```python
from build123d import *

# Parameters (mm, degrees)
SKIZZE1_W                       = 80
SKIZZE1_H                       = 60
AUFSATZ_LINEAR_AUSTRAGEN1_DEPTH = 10
SKIZZE2_W                       = 80
SKIZZE2_H                       = 10
AUFSATZ_LINEAR_AUSTRAGEN2_DEPTH = 10
SKIZZE3_R                       = 11.35
SCHNITT_LINEAR_AUSTRAGEN1_DEPTH = 2.2
SKIZZE4_R                       = 3
SCHNITT_LINEAR_AUSTRAGEN2_DEPTH = 12.2
SKIZZE5_R                       = 2.25
SCHNITT_LINEAR_AUSTRAGEN3_DEPTH = 12.2
SKIZZE6_R                       = 11
SCHNITT_LINEAR_AUSTRAGEN4_DEPTH = 12.2
SKIZZE7_R                       = 1.6
SCHNITT_LINEAR_AUSTRAGEN5_DEPTH = 12.2
SKIZZE8_R                       = 3
SCHNITT_LINEAR_AUSTRAGEN6_DEPTH = 6
FASE1_SIZE                      = 1


with BuildPart() as part:
    # Skizze1 → Aufsatz-Linear austragen1 (new body)
    with BuildSketch(Plane.XY):
        Rectangle(SKIZZE1_W, SKIZZE1_H)
    extrude(amount=AUFSATZ_LINEAR_AUSTRAGEN1_DEPTH)

    # Skizze2 → Aufsatz-Linear austragen2 (add)
    with BuildSketch(Plane.XY.offset(10)):
        with Locations((0, 25)):
            Rectangle(SKIZZE2_W, SKIZZE2_H)
        with Locations((0, -25)):
            Rectangle(SKIZZE2_W, SKIZZE2_H)
    extrude(amount=AUFSATZ_LINEAR_AUSTRAGEN2_DEPTH)

    # Skizze3 → Schnitt-Linear austragen1 (cut)
    with BuildSketch(Plane(origin=(0, 0, 0), x_dir=(-1, 0, 0), z_dir=(0, 0, -1))):
        Circle(SKIZZE3_R)
    extrude(amount=-SCHNITT_LINEAR_AUSTRAGEN1_DEPTH, mode=Mode.SUBTRACT)

    # Skizze4 → Schnitt-Linear austragen2 (cut)
    with BuildSketch(Plane(origin=(0, 0, 2.2), x_dir=(-1, 0, 0), z_dir=(0, 0, -1))):
        Circle(SKIZZE4_R)
    extrude(amount=-SCHNITT_LINEAR_AUSTRAGEN2_DEPTH, mode=Mode.SUBTRACT)

    # Skizze5 → Schnitt-Linear austragen3 (cut)
    with BuildSketch(Plane.XY.offset(20)):
        with Locations((30, 25)):
            Circle(SKIZZE5_R)
        with Locations((-30, 25)):
            Circle(SKIZZE5_R)
        with Locations((-30, -25)):
            Circle(SKIZZE5_R)
        with Locations((30, -25)):
            Circle(SKIZZE5_R)
    extrude(amount=-SCHNITT_LINEAR_AUSTRAGEN3_DEPTH, mode=Mode.SUBTRACT)

    # Skizze6 → Schnitt-Linear austragen4 (cut)
    with BuildSketch(Plane.XY.offset(10)):
        with Locations((-25, 0)):
            Circle(SKIZZE6_R)
        with Locations((25, 0)):
            Circle(SKIZZE6_R)
    extrude(amount=-SCHNITT_LINEAR_AUSTRAGEN4_DEPTH, mode=Mode.SUBTRACT)

    # Skizze7 → Schnitt-Linear austragen5 (cut)
    with BuildSketch(Plane.XY.offset(10)):
        with Locations((-15.55, 15.55)):
            Circle(SKIZZE7_R)
        with Locations((15.55, 15.55)):
            Circle(SKIZZE7_R)
        with Locations((15.55, -15.55)):
            Circle(SKIZZE7_R)
        with Locations((-15.55, -15.55)):
            Circle(SKIZZE7_R)
    extrude(amount=-SCHNITT_LINEAR_AUSTRAGEN5_DEPTH, mode=Mode.SUBTRACT)

    # Skizze8 → Schnitt-Linear austragen6 (cut)
    with BuildSketch(Plane.XY.offset(10)):
        with Locations((-15.55, 15.55)):
            Circle(SKIZZE8_R)
        with Locations((15.55, 15.55)):
            Circle(SKIZZE8_R)
        with Locations((-15.55, -15.55)):
            Circle(SKIZZE8_R)
        with Locations((15.55, -15.55)):
            Circle(SKIZZE8_R)
    extrude(amount=-SCHNITT_LINEAR_AUSTRAGEN6_DEPTH, mode=Mode.SUBTRACT)

    # Fase1
    fase1_edges = [part.edges().sort_by_distance(p)[0] for p in [
        (-36, 0, 0),
        (14, 0, 0),
    ]]
    chamfer(fase1_edges, length=FASE1_SIZE)


solid = part.part
```
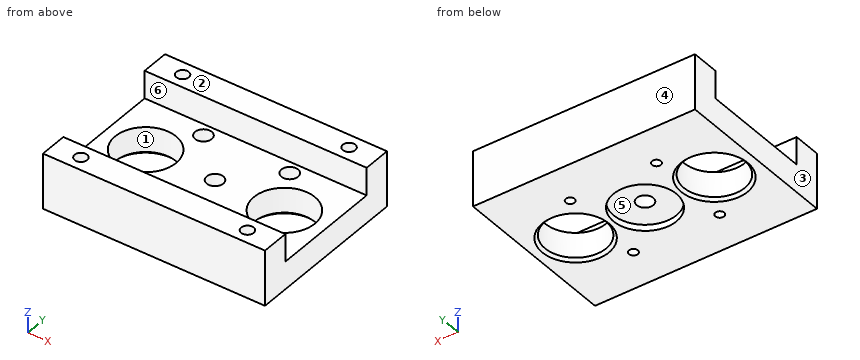
For this review, take the finished solid that the model builds, in its own axes (mm). Face numbers are marked on the shaded views. A direction names the side the tool comes from. Round coordinates to 2 decimals unless told otherwise and drop trailing zeros. Write each loop counter-clockwise with the first axis right and the second up, starting at its lowest first coordinate (ties: lowest second). Pieces come first, ordered by that corner, then holes. Notation, with made-up numbers: (-19.75, 70.25) - (20.25, 70.25) arc R16 cw to (20.25, 81.25) - close; hole circle Ø3 at (-35, 53.25). An arc over 180 degrees is marked (long way). Answer as a JSON object with one key per item and string values.
1. Draft analysis for pull direction X (two halves, no side actions). For the marked faces 1, 2 and 3, state which applies: +X half, -X half, draft (parallel to the pull), parting line (faces both ways), or undercut.
Response values:
{"face 1": "undercut", "face 2": "draft", "face 3": "-X half"}
2. To check wall thickness, follow line 1 along Y through (x, z) = (-30, 11); line 2 along X through (y, z) = (-23, 17); line 3 along X through (y, z) = (-8, 5.5). State the ranges of each line that lie inside material, in increasing order.
Response values:
{"line 1": "y = -30 to -27.25, -22.75 to -20, 20 to 22.75, 27.25 to 30", "line 2": "x = -40 to -31.03, -28.97 to 28.97, 31.03 to 40", "line 3": "x = -40 to -32.55, -17.45 to 17.45, 32.55 to 40"}
3. We need section D-D on y = -15.55. Give the boundary of the cut face in (x, z), then the cut area to 3 significant figures.
Response values:
{"outline": "(-40, 0) - (-17.15, 0) - (-17.15, 4) - (-18.55, 4) - (-18.55, 10) - (-40, 10) - close; (-13.95, 0) - (13.95, 0) - (13.95, 4) - (12.55, 4) - (12.55, 10) - (-12.55, 10) - (-12.55, 4) - (-13.95, 4) - close; (17.15, 0) - (40, 0) - (40, 10) - (18.55, 10) - (18.55, 4) - (17.15, 4) - close", "area": "702 mm2"}
4. Tool access review of the marked faces 4, 5 and 6: name each direction out of +Z, -Z, +X, -X, +Y, -Y from which nothing blocks a thin tool from reaching the whole face with its end or side.
Response values:
{"face 4": "+Z, -Z, +X, -X, +Y", "face 5": "-Z", "face 6": "+Z, +X, -X"}
5. We need section B-B on x = 0. Give the boundary of the cut face in (y, z), then the cut area to 3 significant figures.
Response values:
{"outline": "(-30, 0) - (-11.35, 0) - (-11.35, 2.2) - (-3, 2.2) - (-3, 10) - (-20, 10) - (-20, 20) - (-30, 20) - close; (3, 2.2) - (11.35, 2.2) - (11.35, 0) - (30, 0) - (30, 20) - (20, 20) - (20, 10) - (3, 10) - close", "area": "703 mm2"}
6. We need section A-A on z = 17.25. Give the boundary of the cut face in (x, y).
Response values:
{"outline": "(-40, -30) - (40, -30) - (40, -20) - (-40, -20) - close; (-40, 20) - (40, 20) - (40, 30) - (-40, 30) - close; hole circle Ø4.5 at (-30, -25); hole circle Ø4.5 at (-30, 25); hole circle Ø4.5 at (30, -25); hole circle Ø4.5 at (30, 25)"}
7. For pin 1 Ø6.5 at (x, y) = (-15, 14.5) entering from +Z; pin 2 Ø4 at (x, y) = (-30, -25) entering from +Z, all flat-tipped, find the tip position at first contact; note any pin that passes through.
Response values:
{"pin 1": "stops at z = 10", "pin 2": "stops at z = 7.8"}
8. We need section C-C on y = 0. Give the boundary of the cut face in (x, z).
Response values:
{"outline": "(-40, 0) - (-37, 0) - (-36, 1) - (-36, 10) - (-40, 10) - close; (-14, 1) - (-13, 0) - (-11.35, 0) - (-11.35, 2.2) - (-3, 2.2) - (-3, 10) - (-14, 10) - close; (3, 2.2) - (11.35, 2.2) - (11.35, 0) - (13, 0) - (14, 1) - (14, 10) - (3, 10) - close; (36, 1) - (37, 0) - (40, 0) - (40, 10) - (36, 10) - close"}
